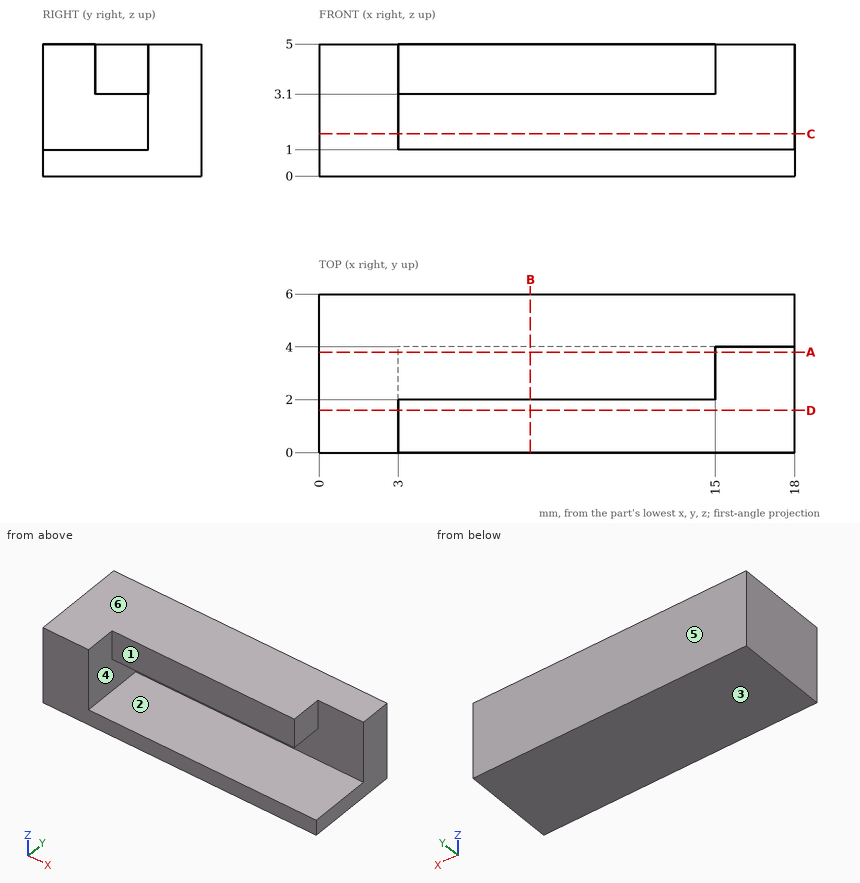
Input: dimensioned drawing with shaded views. Units: mm. Origin: part minimum x, y, z. A direction names the side the tool comes from. Coordinates: 2 decimals unless noted, no trailing zeros. Order: outer loops, then holes, each group sorted by start corner. A loop starts at its lowest first (then second) coordinate and runs counter-clockwise, first axis right, second up. Notation, with made-up numbers: (63, 36) - (89, 36) arc R21 cw to (89, 51) - close; hole circle Ø3 at (48.5, 64.5). An arc over 180 degrees is marked (long way). Put each result on its own line as item: value.
1. Contact query for flat-ended pins moving along their axis: pin 1 Ø1 at (x, z) = (7.5, 4.5) entering from -Y; pin 2 Ø2 at (y, z) = (2, 2.5) entering from +X. Output: stop coordinate, or through.
Report:
pin 1: stops at y = 2
pin 2: stops at x = 15
2. Cut plane B-B on x = 8. Return the cut outline in (y, z).
Report:
outline: (0, 0) - (6, 0) - (6, 5) - (2, 5) - (2, 3.1) - (4, 3.1) - (4, 1) - (0, 1) - close
3. Cut plane C-C on z = 1.6. Return the cut outline in (x, y), then the cut area to 3 significant figures.
Report:
outline: (0, 0) - (3, 0) - (3, 4) - (18, 4) - (18, 6) - (0, 6) - close
area: 48.0 mm2
4. Cut plane A-A on y = 3.8. Return the cut outline in (x, z).
Report:
outline: (0, 0) - (18, 0) - (18, 1) - (3, 1) - (3, 3.1) - (15, 3.1) - (15, 5) - (0, 5) - close
5. Line query: line 1 along Z through (x, y) = (12.25, 2.6); line 2 along Z through (x, y) = (7.5, 1.05); line 3 along Y through (x, z) = (12.5, 1.9). Output: solid intervals per line, ascending.
Report:
line 1: z = 0 to 1, 3.1 to 5
line 2: z = 0 to 1
line 3: y = 4 to 6
6. Reachability of the marked faces 1, 2 and 3 from +Z, -Z, +X, -X, +Y, -Y: full face, straight path, thin tool, end or side. Return the list, or none.
Report:
face 1: +Z, +X, -Y
face 2: +X, -Y
face 3: -Z, +X, -X, +Y, -Y
7. Cut plane D-D on y = 1.6. Return the cut outline in (x, z).
Report:
outline: (0, 0) - (18, 0) - (18, 1) - (3, 1) - (3, 5) - (0, 5) - close
8. Draft query along Z for the marked faces 4, 5 and 6. Return one class per face: pulls with the +Z half, pulls with the -Z half, needs draft (parallel to the pull), parting line crosses it, or undercut.
Report:
face 4: undercut
face 5: needs draft
face 6: pulls with the +Z half
